Design review of the part shown in the three views and the two pictorial views. Dimensions are in mm from the part's minimum x, y and z. Give positions to 0.01 mm unless a question says otherwise; leave off trailing zeros. Order: outer loops, then holes, each group sorted by start corner. A loop starts at its lowest first (then second) coordinate and runs counter-clockwise, first axis right, second up. Notation, with made-up numbers: M 45.25,46 L 56.25,46 A26 ccw 56.25,81 Z; hole C 17,-32.5 d4. An arc over 180 degrees is marked long. Answer as a JSON object with one key per item and string values.
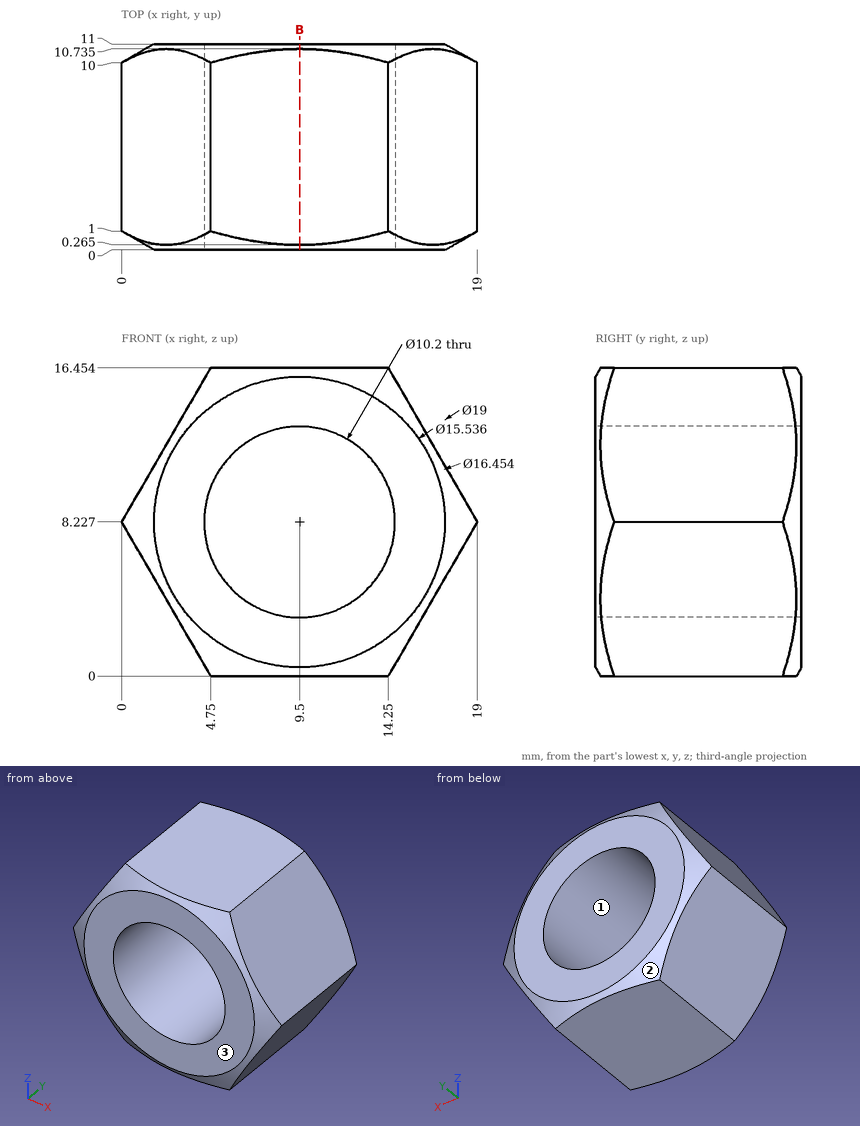
(1) To check wall thickness, follow L1, parallel to Z at x = 9.5, y = 5.5 (1 decimal); L2, parallel to X at y = 0.5, z = 11; L3, parallel to X at y = 4.5, z = 4.5. State the ranges of each line that lie inside material, in increasing order. Write a range as from..to.
Checked values:
{"L1": "z = 0..3.1, 13.3..16.5", "L2": "x = 1.6..5.22, 13.78..17.4", "L3": "x = 2.15..6.02, 12.98..16.85"}
(2) Draft analysis for pull direction Z (two halves, no side actions). For the marked faces 1, 2 and 3, state which applies: +Z half, -Z half, draft (parallel to the pull), parting line (faces both ways), or undercut.
Checked values:
{"face 1": "undercut", "face 2": "parting line", "face 3": "draft"}
(3) We need section B-B (x = 9.5). Write out the cut boundary in (y, z) (1 decimal).
Checked values:
{"outline": "M 0,0.5 L 0.3,0 L 10.7,0 L 11,0.5 L 11,3.1 L 0,3.1 Z; M 0,13.3 L 11,13.3 L 11,16 L 10.7,16.5 L 0.3,16.5 L 0,16 Z"}
(4) Insertion check: pin 1 (1 mm diameter, centred on y = 7, z = 6, fed in from +X); pin 2 (4 mm diameter, centred on y = 8, z = 3.5, fed in from -X) (1 decimal). Each pin has a flat end and moves straight along its axis. Give the tip position at first contact, or say it passes through.
Checked values:
{"pin 1": "stops at x = 18", "pin 2": "stops at x = 1.6"}
